from build123d import *

# Parameters (mm, degrees)
SKETCH1_W                     = 10
SKETCH1_H                     = 1.5
BASE_BUTTERFLY_BLOCKS_DEPTH   = 5
SKETCH1_W_2                   = 1.5
SKETCH1_H_2                   = 10
BASE_BUTTERFLY_BLOCKS_2_DEPTH = 5
BASE_BUTTERFLY_BLOCKS_3_DEPTH = 5
BASE_BUTTERFLY_BLOCKS_4_DEPTH = 5
BASE_BUTTERFLY_BLOCKS_5_DEPTH = 5
BASE_BUTTERFLY_BLOCKS_6_DEPTH = 5
BASE_BUTTERFLY_FLEXURES_DEPTH = 2.5
SKETCH3_W                     = 10
SKETCH3_H                     = 10
BOSS_EXTRUDE4_DEPTH           = 10
BOSS_EXTRUDE5_DEPTH           = 10


with BuildPart() as part:
    # Sketch1 → base_butterfly_blocks (new, symmetric)
    with BuildSketch(Plane(origin=(0, 0, 0), x_dir=(1, 0, 0), z_dir=(0, 1, 0))):
        with Locations((0, -9.410254038)):
            Rectangle(SKETCH1_W, SKETCH1_H)
    extrude(amount=BASE_BUTTERFLY_BLOCKS_DEPTH, both=True)



with BuildPart() as body_2:
    # Sketch1 → base_butterfly_blocks 2 (new, symmetric)
    with BuildSketch(Plane(origin=(0, 0, 0), x_dir=(1, 0, 0), z_dir=(0, 1, 0))):
        with Locations((-9.410254038, 0)):
            Rectangle(SKETCH1_W_2, SKETCH1_H_2)
    extrude(amount=BASE_BUTTERFLY_BLOCKS_2_DEPTH, both=True)


with BuildPart() as body_3:
    # Sketch1 → base_butterfly_blocks 3 (new, symmetric)
    with BuildSketch(Plane(origin=(0, 0, 0), x_dir=(1, 0, 0), z_dir=(0, 1, 0))):
        with Locations((0, 9.410254038)):
            Rectangle(SKETCH1_W, SKETCH1_H)
    extrude(amount=BASE_BUTTERFLY_BLOCKS_3_DEPTH, both=True)


with BuildPart() as body_4:
    # Sketch1 → base_butterfly_blocks 4 (new, symmetric)
    with BuildSketch(Plane(origin=(0, 0, 0), x_dir=(1, 0, 0), z_dir=(0, 1, 0))):
        with Locations((9.410254038, 0)):
            Rectangle(SKETCH1_W_2, SKETCH1_H_2)
    extrude(amount=BASE_BUTTERFLY_BLOCKS_4_DEPTH, both=True)


with BuildPart() as body_5:
    # Sketch1 → base_butterfly_blocks 5 (new, symmetric)
    with BuildSketch(Plane(origin=(0, 0, 0), x_dir=(1, 0, 0), z_dir=(0, 1, 0))):
        with BuildLine():
            Line((-1.971217842, 0.338083152), (-2.464022303, 0.42260394))
            ThreePointArc((-2.464022303, 0.42260394), (0, 2.5), (2.464022303, 0.42260394))
            Line((2.464022303, 0.42260394), (1.971217842, 0.338083152))
            ThreePointArc((1.971217842, 0.338083152), (0, 2), (-1.971217842, 0.338083152))
        make_face()
    extrude(amount=BASE_BUTTERFLY_BLOCKS_5_DEPTH, both=True)


with BuildPart() as body_6:
    # Sketch1 → base_butterfly_blocks 6 (new, symmetric)
    with BuildSketch(Plane(origin=(0, 0, 0), x_dir=(1, 0, 0), z_dir=(0, 1, 0))):
        with BuildLine():
            ThreePointArc((-1.971217842, -0.338083152), (0, -2), (1.971217842, -0.338083152))
            Line((1.971217842, -0.338083152), (2.464022303, -0.42260394))
            ThreePointArc((2.464022303, -0.42260394), (0, -2.5), (-2.464022303, -0.42260394))
            Line((-2.464022303, -0.42260394), (-1.971217842, -0.338083152))
        make_face()
    extrude(amount=BASE_BUTTERFLY_BLOCKS_6_DEPTH, both=True)


with BuildPart() as part_1:
    add(part.part)

    add(body_2.part)  # base_butterfly_flexures merges body 2

    add(body_3.part)  # base_butterfly_flexures merges body 3

    add(body_4.part)  # base_butterfly_flexures merges body 4

    add(body_5.part)  # base_butterfly_flexures merges body 5

    add(body_6.part)  # base_butterfly_flexures merges body 6
    # Sketch1<4> → base_butterfly_flexures (add, symmetric)
    with BuildSketch(Plane(origin=(0, 0, 0), x_dir=(1, 0, 0), z_dir=(0, 1, 0))):
        with BuildLine():
            Line((-8.660254038, 5), (-8.660254038, 4))
            Line((-8.660254038, 4), (-2.464022303, 0.42260394))
            ThreePointArc((-2.464022303, 0.42260394), (-2.351224133, 0.84955581), (-2.165063509, 1.25))
            Line((-2.165063509, 1.25), (-8.660254038, 5))
        make_face()
        with BuildLine():
            Line((-5, 8.660254038), (-1.25, 2.165063509))
            ThreePointArc((-1.25, 2.165063509), (-0.84955581, 2.351224133), (-0.42260394, 2.464022303))
            Line((-0.42260394, 2.464022303), (-4, 8.660254038))
            Line((-4, 8.660254038), (-5, 8.660254038))
        make_face()
        with BuildLine():
            Line((4, 8.660254038), (0.42260394, 2.464022303))
            ThreePointArc((0.42260394, 2.464022303), (0.84955581, 2.351224133), (1.25, 2.165063509))
            Line((1.25, 2.165063509), (5, 8.660254038))
            Line((5, 8.660254038), (4, 8.660254038))
        make_face()
        with BuildLine():
            Line((2.464022303, 0.42260394), (8.660254038, 4))
            Line((8.660254038, 4), (8.660254038, 5))
            Line((8.660254038, 5), (2.165063509, 1.25))
            ThreePointArc((2.165063509, 1.25), (2.351224133, 0.84955581), (2.464022303, 0.42260394))
        make_face()
        with BuildLine():
            ThreePointArc((2.464022303, -0.42260394), (2.351224133, -0.84955581), (2.165063509, -1.25))
            Line((2.165063509, -1.25), (8.660254038, -5))
            Line((8.660254038, -5), (8.660254038, -4))
            Line((8.660254038, -4), (2.464022303, -0.42260394))
        make_face()
        with BuildLine():
            ThreePointArc((1.25, -2.165063509), (0.84955581, -2.351224133), (0.42260394, -2.464022303))
            Line((0.42260394, -2.464022303), (4, -8.660254038))
            Line((4, -8.660254038), (5, -8.660254038))
            Line((5, -8.660254038), (1.25, -2.165063509))
        make_face()
        with BuildLine():
            ThreePointArc((-0.42260394, -2.464022303), (-0.84955581, -2.351224133), (-1.25, -2.165063509))
            Line((-1.25, -2.165063509), (-5, -8.660254038))
            Line((-5, -8.660254038), (-4, -8.660254038))
            Line((-4, -8.660254038), (-0.42260394, -2.464022303))
        make_face()
        with BuildLine():
            Line((-8.660254038, -5), (-2.165063509, -1.25))
            ThreePointArc((-2.165063509, -1.25), (-2.351224133, -0.84955581), (-2.464022303, -0.42260394))
            Line((-2.464022303, -0.42260394), (-8.660254038, -4))
            Line((-8.660254038, -4), (-8.660254038, -5))
        make_face()
    extrude(amount=BASE_BUTTERFLY_FLEXURES_DEPTH, both=True)

    # Sketch3 → Boss-Extrude4 (add)
    with BuildSketch(Plane(origin=(0, 0, -10.160254038), x_dir=(-1, 0, 0), z_dir=(0, 0, -1))):
        Rectangle(SKETCH3_W, SKETCH3_H)
    extrude(amount=BOSS_EXTRUDE4_DEPTH)

    # Sketch4 → Boss-Extrude5 (add)
    with BuildSketch(Plane(origin=(0, 5, 0), x_dir=(1, 0, 0), z_dir=(0, 1, 0))):
        with BuildLine():
            ThreePointArc((-5, 20.160254038), (0, 25.160254038), (5, 20.160254038))
            Line((5, 20.160254038), (-5, 20.160254038))
        make_face()
    extrude(amount=-BOSS_EXTRUDE5_DEPTH)


solid = part_1.part
Design review of the part built by this model. Coordinates are the model's own, in mm. A direction names the side the tool comes from. Coordinates: 2 decimals unless noted, no trailing zeros. Order: outer loops, then holes, each group sorted by start corner. A loop starts at its lowest first (then second) coordinate and runs counter-clockwise, first axis right, second up. Notation, with made-up numbers: M -27.75,-18.75 L 10.25,-18.75 A32 ccw 10.25,20.25 Z; hole C 80.5,87 d2. An arc over 180 degrees is marked long. Use a Markdown table: item, result.
(1) For P1, Ø3.5, axis at x = 2.5, z = -6, coming from the +Y side; P2, Ø1, axis at x = 6.5, z = -3.5, coming from the -Y side; P3, Ø1.6, axis at x = -9.5, y = 0, coming from the +Z side, all flat-tipped, find the tip position at first contact; note any pin that passes through.
Worked answers:
| item | result |
|---|---|
| P1 | stops at y = 2.5 |
| P2 | stops at y = -2.5 |
| P3 | stops at z = 5 |
(2) For faces 3 (the cylindrical face through (0, 0.1, -2.5)), 4 (the flat face through (3.151, -0.035, 5.458)), 5 (the flat face through (5.4, 2.5, -2.7)), 6 (the flat face through (-2.7, -2.5, 5.4)), list the 3-axis set-ups (+Z, -Z, +X, -X, +Y, -Y) from which the entire face can be reached by the end or side of a thin tool; tool diameter is ignored.
Worked answers:
| item | result |
|---|---|
| face 3 | none |
| face 4 | +Y, -Y |
| face 5 | +Y |
| face 6 | -Y |
(3) Add section D-D (y = 2). Count the separate pieces of the cut face and the enclosed holes in it, then the cut area to 3 significant figures.
Worked answers:
| item | result |
|---|---|
| separate pieces | 1 |
| enclosed holes | 3 |
| area | 256 mm2 |
(4) Add section A-A (x = 0). Give the boundary of the cut face in (y, z), then the cut area to 3 significant figures.
Worked answers:
| item | result |
|---|---|
| outline | M -5,-25.16 L 5,-25.16 L 5,-8.66 L -5,-8.66 Z; M -5,-2.5 L 5,-2.5 L 5,-2 L -5,-2 Z; M -5,2 L 5,2 L 5,2.5 L -5,2.5 Z; M -5,8.66 L 5,8.66 L 5,10.16 L -5,10.16 Z |
| area | 190 mm2 |
(5) Wall thickness on probe 1 along Z at (x, y) = (-4.5, 0.75); probe 2 along X at (y, z) = (3.5, -10): over which ranges is each line inside the solid? List them lowest first.
Worked answers:
| item | result |
|---|---|
| probe 1 | z = -22.34 to -7.79, -2.6 to -1.6, 1.6 to 2.6, 7.79 to 10.16 |
| probe 2 | x = -5 to 5 |
(6) Add section B-B (y = 3.75). Give the boundary of the cut face in (x, z).
Worked answers:
| item | result |
|---|---|
| outline | M -10.16,-5 L -8.66,-5 L -8.66,5 L -10.16,5 Z; M -5,-20.16 A5 ccw 5,-20.16 L 5,-8.66 L -5,-8.66 Z; M -5,8.66 L 5,8.66 L 5,10.16 L -5,10.16 Z; M -2.46,-0.42 A2.5 ccw 2.46,-0.42 L 1.97,-0.34 A2 cw -1.97,-0.34 Z; M -2.46,0.42 L -1.97,0.34 A2 cw 1.97,0.34 L 2.46,0.42 A2.5 ccw Z; M 8.66,-5 L 10.16,-5 L 10.16,5 L 8.66,5 Z |
(7) Draft analysis for pull direction Z (two halves, no side actions). For faces 1 (the flat face through (-0.171, 5, -2.145)), 2 (the flat face through (-2.24, -0.04, 5.61)), state which applies: released by +Z, released by -Z, zero draft, split by the parting line, or undercut.
Worked answers:
| item | result |
|---|---|
| face 1 | zero draft |
| face 2 | undercut |
(8) Add section C-C (z = 3.5). Give the boundary of the cut face in (x, y).
Worked answers:
| item | result |
|---|---|
| outline | M -10.16,-5 L -8.66,-5 L -8.66,5 L -10.16,5 Z; M -7.79,-2.5 L -6.06,-2.5 L -6.06,2.5 L -7.79,2.5 Z; M -2.02,-2.5 L -1.02,-2.5 L -1.02,2.5 L -2.02,2.5 Z; M 1.02,-2.5 L 2.02,-2.5 L 2.02,2.5 L 1.02,2.5 Z; M 6.06,-2.5 L 7.79,-2.5 L 7.79,2.5 L 6.06,2.5 Z; M 8.66,-5 L 10.16,-5 L 10.16,5 L 8.66,5 Z |
